from build123d import *

# Parameters (mm, degrees)
F0_R     = 12.3
F0_R_2   = 10.9
F0_R_3   = 7.1
F0_R_4   = 5.7
F0_R_5   = 2.9
F0_R_6   = 1.9
F1_DEPTH = 2
F2_DEPTH = 10
F3_DEPTH = 25
F4_W     = 2.2
F4_H     = 35
F5_DEPTH = 12.301
F6_SIZE  = 1.2


with BuildPart() as f1:
    # F0 (on Top) → F1 (new body)
    with BuildSketch(Plane.XY):
        Circle(F0_R)
        Circle(F0_R_2, mode=Mode.SUBTRACT)
        Circle(F0_R_2)
        Circle(F0_R_3, mode=Mode.SUBTRACT)
        Circle(F0_R_3)
        Circle(F0_R_4, mode=Mode.SUBTRACT)
        Circle(F0_R_4)
        Circle(F0_R_5, mode=Mode.SUBTRACT)
        Circle(F0_R_5)
        Circle(F0_R_6, mode=Mode.SUBTRACT)
    extrude(amount=-F1_DEPTH)

    # F0 (on Top) → F2 (join)
    with BuildSketch(Plane.XY):
        Circle(F0_R_3)
        Circle(F0_R_4, mode=Mode.SUBTRACT)
        Circle(F0_R_5)
        Circle(F0_R_6, mode=Mode.SUBTRACT)
    extrude(amount=-F2_DEPTH)

    # F0 (on Top) → F3 (join)
    with BuildSketch(Plane.XY):
        Circle(F0_R)
        Circle(F0_R_2, mode=Mode.SUBTRACT)
    extrude(amount=F3_DEPTH)

    # F4 (on Front) → F5 (cut, through all)
    with BuildSketch(Plane.XZ):
        with Locations((0, 7.5)):
            Rectangle(F4_W, F4_H)
    extrude(amount=-F5_DEPTH, mode=Mode.SUBTRACT)

    # F6
    f6_edges = [f1.edges().sort_by_distance(p)[0] for p in [
        (0, -7.1, -2),
    ]]
    chamfer(f6_edges, length=F6_SIZE)


solid = f1.part
The listing builds one solid part. Answer for the finished solid, in the listing's coordinates (mm). A direction names the side the tool comes from. Coordinates: 2 decimals unless noted, no trailing zeros. Write each loop counter-clockwise with the first axis right and the second up, starting at its lowest first coordinate (ties: lowest second). Pieces come first, ordered by that corner, then holes. Notation, with made-up numbers: (-27, 9.25) - (3, 9.25) arc R20 ccw to (3, 46.25) - close; hole circle Ø1 at (27, -21.5). An arc over 180 degrees is marked (long way). Return JSON: item names as keys, results as strings.
1. Each of these flat-tipped pins is pushed along its axis until it touches: pin 1 Ø3 at (x, z) = (3.5, 3) entering from +Y; pin 2 Ø5.5 at (y, z) = (9, 10) entering from -X; pin 3 Ø5 at (y, z) = (-7.5, 17) entering from +X; pin 4 Ø3 at (x, y) = (0, 0) entering from -Z. Where does it stop, or does it pass through?
Final values:
{"pin 1": "y = 12.14", "pin 2": "x = -10.59", "pin 3": "x = 11.24", "pin 4": "through"}
2. Which of the six approach directions +Z, -Z, +X, -X, +Y, -Y give full straight-line access (tool end or side, diameter ignored) to faces 1 (the face through (-1.1, 7.7, -0.4)), 2 (the face through (3, -8, -2)), 3 (the face through (-0.2, -2.3, 0))?
Final values:
{"face 1": "+Z, -Z, +Y", "face 2": "-Z", "face 3": "+Z"}
3. The part is cut by section D-D on x = 9.5. Determine the outline of the cut face in (y, z).
Final values:
{"outline": "(-7.81, -2) - (7.81, -2) - (7.81, 25) - (5.34, 25) - (5.34, 0) - (-5.34, 0) - (-5.34, 25) - (-7.81, 25) - close"}
4. The part is cut by section A-A on y = 0. Determine the outline of the cut face in (x, z).
Final values:
{"outline": "(-12.3, -2) - (-8.3, -2) - (-7.1, -3.2) - (-7.1, -10) - (-5.7, -10) - (-5.7, -2) - (-2.9, -2) - (-2.9, -10) - (-1.9, -10) - (-1.9, 0) - (-10.9, 0) - (-10.9, 25) - (-12.3, 25) - close; (1.9, -10) - (2.9, -10) - (2.9, -2) - (5.7, -2) - (5.7, -10) - (7.1, -10) - (7.1, -3.2) - (8.3, -2) - (12.3, -2) - (12.3, 25) - (10.9, 25) - (10.9, 0) - (1.9, 0) - close"}
5. The part is cut by section B-B on x = 0. Determine the outline of the cut face in (y, z), then the cut area to 3 significant figures.
Final values:
{"outline": "(-12.3, -2) - (-8.3, -2) - (-7.1, -3.2) - (-7.1, -10) - (-5.7, -10) - (-5.7, -2) - (-2.9, -2) - (-2.9, -10) - (-1.9, -10) - (-1.9, 0) - (-10.9, 0) - (-10.9, 25) - (-12.3, 25) - close", "area": "75.7 mm^2"}
6. For a pull along Y with two mould halves and no side action, classify faces 4 (the face through (-0.07, -1.9, -4.93)), 5 (the face through (-2, -11, 25)), 6 (the face through (-0.46, -10.89, 12.32)), 7 (the face through (-0.308, -7.302, -2.992)) as +Y half, -Y half, draft (parallel to the pull), parting line (faces both ways), or undercut.
Final values:
{"face 4": "undercut", "face 5": "draft", "face 6": "undercut", "face 7": "parting line"}
7. Consider line 1 along X through (y, z) = (0, -6); line 2 along X through (y, z) = (0, 17.5); line 3 along Y through (x, z) = (0, -4.75). Determine where each line is inside the solid, lowest interval first.
Final values:
{"line 1": "-7.1 to -5.7, -2.9 to -1.9, 1.9 to 2.9, 5.7 to 7.1", "line 2": "-12.3 to -10.9, 10.9 to 12.3", "line 3": "-7.1 to -5.7, -2.9 to -1.9"}
8. The part is cut by section C-C on z = 1. Determine the outline of the cut face in (x, y).
Final values:
{"outline": "(-1.1, 10.84) - (-1.1, 12.25) arc R12.3 ccw (long way) to (1.1, 12.25) - (1.1, 10.84) arc R10.9 cw (long way) to start"}
